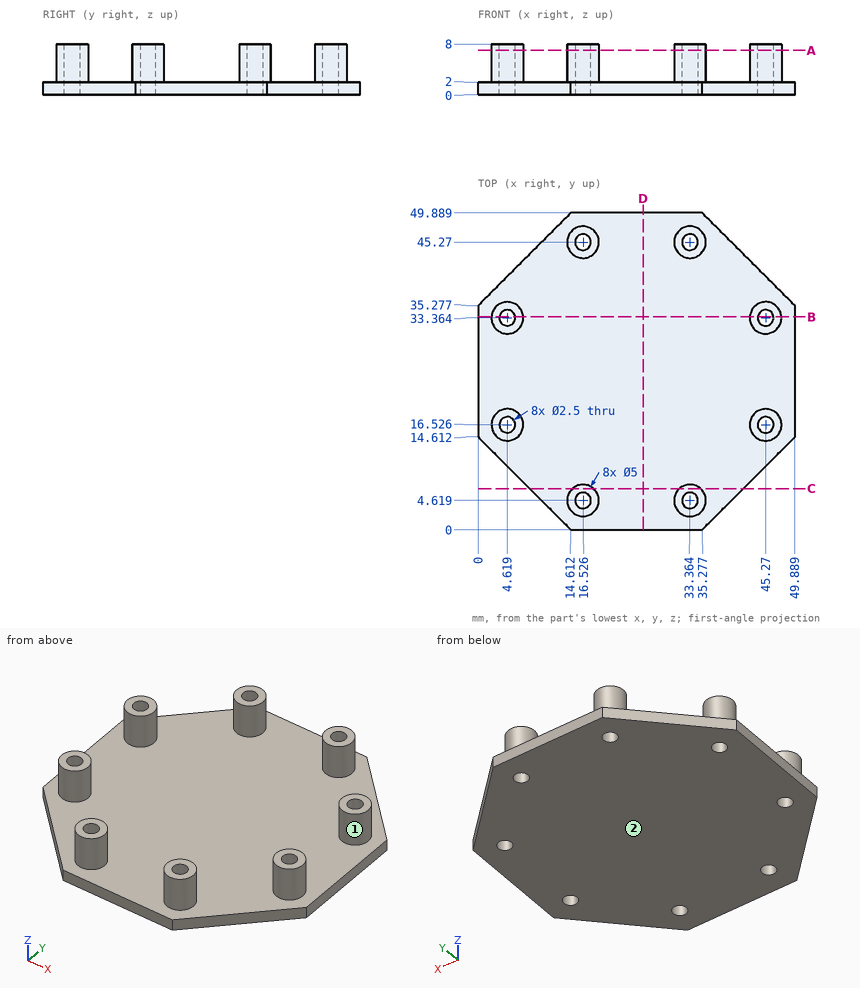
Study the drawing (mm; zero at the part's minimum x, y, z) and answer. Coordinates: 2 decimals unless noted, no trailing zeros. Write each loop counter-clockwise with the first axis right and the second up, starting at its lowest first coordinate (ties: lowest second). Pieces come first, ordered by that corner, then holes. Notation, with made-up numbers: (57, -28.75) -> (98, -28.75) arc R30 cw to (98, 9.25) -> close; hole circle Ø9 at (47, -2). An arc over 180 degrees is marked (long way). Write item = value, one per line.
(1) Section B-B on y = 33.5 is taken. Write down the section's boundary in (x, z) (1 decimal), plus the area to 3 significant figures.
From the geometry:
outline = (0, 0) -> (3.4, 0) -> (3.4, 8) -> (2.1, 8) -> (2.1, 2) -> (0, 2) -> close; (5.9, 0) -> (44, 0) -> (44, 8) -> (42.8, 8) -> (42.8, 2) -> (7.1, 2) -> (7.1, 8) -> (5.9, 8) -> close; (46.5, 0) -> (49.9, 0) -> (49.9, 2) -> (47.8, 2) -> (47.8, 8) -> (46.5, 8) -> close
area = 120 mm2
(2) Given pin 1 Ø2 at (x, y) = (4.62, 33.36) entering from +Z; pin 2 Ø1.5 at (x, z) = (42.5, 3) entering from -Y (1 decimal); pin 3 Ø1.5 at (y, z) = (9.5, 1.5) entering from -X, each flat-ended and moving along its own axis, determine where each tip first touches the part or whether it passes through.
From the geometry:
pin_1 = through
pin_2 = 15.1
pin_3 = 4.36
(3) Straight lines are drawn through the part: L1, parallel to X at y = 16.5, z = 2.25; L2, parallel to X at y = 33, z = 7 (1 decimal); L3, parallel to Z at x = 11, y = 29. For each, find the intervals that lie inside material, in ascending order. Write a range as from..to.
From the geometry:
L1 = 2.12..3.37, 5.87..7.12, 42.77..44.02, 46.52..47.77
L2 = 2.1..3.4, 5.8..7.1, 42.8..44.1, 46.5..47.7
L3 = 0..2
(4) For a pull along Y with two mould halves and no side action, classify the marked faces 1 and 2 as +Y half, -Y half, draft (parallel to the pull), parting line (faces both ways), or undercut.
From the geometry:
face_1 = undercut
face_2 = draft
(5) Section D-D on x = 26 is taken. Write down the section's boundary in (y, z).
From the geometry:
outline = (0, 0) -> (49.89, 0) -> (49.89, 2) -> (0, 2) -> close
(6) Section A-A on z = 7 is taken. Count the separate pieces of the cut face and the enclosed holes in it, plus the area to 3 significant figures.
From the geometry:
separate_pieces = 8
enclosed_holes = 8
area = 118 mm2
(7) Section C-C on y = 6.5 is taken. Write down the section's boundary in (x, z).
From the geometry:
outline = (8.11, 0) -> (41.78, 0) -> (41.78, 2) -> (35.01, 2) -> (35.01, 8) -> (31.72, 8) -> (31.72, 2) -> (18.17, 2) -> (18.17, 8) -> (14.88, 8) -> (14.88, 2) -> (8.11, 2) -> close
